from build123d import *

# Parameters (mm, degrees)
SKETCH_1_W                 = 140
SKETCH_1_H                 = 77.4
EXTRUDE_1_DEPTH            = 15
SKETCH_6_R                 = 10.5
CUT_EXTRUDE_4_DEPTH        = 161.315345491
M5X0_8_1_D                 = 4.2
M5X0_8_1_DEPTH             = 16
M5X0_8_1_TIP               = 1.2618073
SKETCH_9_R                 = 10
CUT_EXTRUDE_6_DEPTH        = 161.67283529
M5X0_8_2_D                 = 4.2
HOLE_WIZARD_M3_1_D         = 3.4
M6X1_0_START               = -77.4
M6X1_0_3_OUTLINE_R         = 2.5
M6X1_0_3_DEPTH             = 77.4
HOLE_WIZARD_M3_2_OUTLINE_R = 1.7
HOLE_WIZARD_M3_2_DEPTH     = 15
M7X1_0_4_OUTLINE_W         = 3
M7X1_0_4_OUTLINE_H         = 20.46087378
CUT_EXTRUDE_7_REACH        = 137.336
SKETCH_27_R                = 3


# Read off the part's stored shape, not the designer's step: M6x1.0 ねじ穴3, M3 すきま穴2, M7x1.0 ねじ穴4
with BuildPart() as part:
    # ｽｹｯﾁ1 → ﾎﾞｽ - 押し出し1 (new body)
    with BuildSketch(Plane(origin=(0, 0, 0), x_dir=(1, 0, 0), z_dir=(0, 1, 0))):
        with Locations((70, 38.7)):
            Rectangle(SKETCH_1_W, SKETCH_1_H)
    extrude(amount=EXTRUDE_1_DEPTH)

    # ｽｹｯﾁ6 → ｶｯﾄ - 押し出し4 (cut, through all)
    with BuildSketch(Plane(origin=(0, 10.5, 0), x_dir=(1, 0, 0), z_dir=(0, 1, 0))):
        with Locations(Location((110, 30, 0), (0, 0, 270))):
            Circle(SKETCH_6_R)
    extrude(amount=-CUT_EXTRUDE_4_DEPTH, mode=Mode.SUBTRACT)

    # M5x0.8 ねじ穴1
    with Locations(Plane(origin=(140, 0, 0), x_dir=(0, 0, -1), z_dir=(1, 0, 0))):
        with Locations((10.4, 7.5), (67.4, 7.5)):
            Hole(M5X0_8_1_D / 2, depth=M5X0_8_1_DEPTH)
            with Locations((0, 0, -(M5X0_8_1_DEPTH + M5X0_8_1_TIP / 2))):  # 118° drill point
                Cone(0, M5X0_8_1_D / 2, M5X0_8_1_TIP, mode=Mode.SUBTRACT)

    # ｽｹｯﾁ9 → ｶｯﾄ - 押し出し6 (cut, through all)
    with BuildSketch(Plane(origin=(0, 15, 0), x_dir=(1, 0, 0), z_dir=(0, 1, 0))):
        with Locations(Location((30, 30, 0), (0, 0, 270))):
            Circle(SKETCH_9_R)
    extrude(amount=-CUT_EXTRUDE_6_DEPTH, mode=Mode.SUBTRACT)

    # M5x0.8 ねじ穴2 (through all)
    with Locations(Plane(origin=(0, 15, 0), x_dir=(1, 0, 0), z_dir=(0, 1, 0))):
        with Locations((42.991460674, 42.458810119), (17.272077939, 42.727922061), (42.727922061, 17.272077939), (17.541189881, 17.008539326)):
            Hole(M5X0_8_2_D / 2)

    # M3 すきま穴1 (through all)
    with Locations(Plane(origin=(0, 15, 0), x_dir=(1, 0, 0), z_dir=(0, 1, 0))):
        with Locations((119.899494937, 39.899494937), (119.899494937, 20.100505063), (100.100505063, 20.100505063), (100.100505063, 39.899494937)):
            Hole(HOLE_WIZARD_M3_1_D / 2)

    # M6x1.0 ねじ穴3 outline → M6x1.0 ねじ穴3 (cut)
    with BuildSketch(Plane.XY.offset(M6X1_0_START)):
        with Locations((84.5, 7.5)):
            Circle(M6X1_0_3_OUTLINE_R)
    extrude(amount=M6X1_0_3_DEPTH, mode=Mode.SUBTRACT)

    # M3 すきま穴2 outline → M3 すきま穴2 (cut)
    with BuildSketch(Plane(origin=(0, 0, 0), x_dir=(1, 0, 0), z_dir=(0, 1, 0))):
        with Locations((92.5, 73.4)):
            Circle(HOLE_WIZARD_M3_2_OUTLINE_R)
        with Locations((127.5, 73.4)):
            Circle(HOLE_WIZARD_M3_2_OUTLINE_R)
        with Locations((92.5, 4)):
            Circle(HOLE_WIZARD_M3_2_OUTLINE_R)
        with Locations((127.5, 4)):
            Circle(HOLE_WIZARD_M3_2_OUTLINE_R)
    extrude(amount=HOLE_WIZARD_M3_2_DEPTH, mode=Mode.SUBTRACT)

    # M7x1.0 ねじ穴4 outline → M7x1.0 ねじ穴4 (revolve, cut)
    with BuildSketch(Plane(origin=(0, 7.5, -30), x_dir=(0, 1, 0), z_dir=(0, 0, -1))):
        with Locations((1.5, 10.23043689)):
            Rectangle(M7X1_0_4_OUTLINE_W, M7X1_0_4_OUTLINE_H)
    revolve(axis=Axis((0, 7.5, -30), (1, 0, 0)), mode=Mode.SUBTRACT)

    # ｽｹｯﾁ27 → ｶｯﾄ - 押し出し7 (cut, up to next)
    with BuildSketch(Plane.ZY.offset(-30), mode=Mode.PRIVATE) as cut_extrude_7_sk1:
        with Locations((-30, 7.5)):
            Circle(SKETCH_27_R)
    cut_extrude_7_tool1 = extrude(cut_extrude_7_sk1.sketch, amount=-CUT_EXTRUDE_7_REACH, mode=Mode.PRIVATE) & part.part
    add(cut_extrude_7_tool1.solids().sort_by_distance((30, 7.5, -30))[0], mode=Mode.SUBTRACT)


solid = part.part
Build history of the part. All positions in model axes, mm. A direction names the side the tool comes from. Round coordinates to 2 decimals unless told otherwise and drop trailing zeros. Write each loop counter-clockwise with the first axis right and the second up, starting at its lowest first coordinate (ties: lowest second). Pieces come first, ordered by that corner, then holes. Notation, with made-up numbers: M 20,60 L 59,60 A20 ccw 59,79 Z; hole C 16.25,-14.5 d10. An arc over 180 degrees is marked long. Answer in a Markdown table with one row per item.
1. Probe L1, parallel to X at y = 1.25, z = -42.5; L2, parallel to X at y = 12, z = -4; L3, parallel to X at y = 8.75, z = -73.4. List the from-to ranges inside material, lowest first. Write a range as [from, to].
Geometry check:
| item | result |
|---|---|
| L1 | [0, 15.18], [19.36, 40.89], [45.09, 140] |
| L2 | [0, 90.8], [94.2, 125.8], [129.2, 140] |
| L3 | [0, 82.33], [86.67, 90.8], [94.2, 125.8], [129.2, 140] |
2. Saw through at B-B (z = -4). List the corners of the cut face in (x, y), and give its area (3 significant figures).
Geometry check:
| item | result |
|---|---|
| outline | M 0,0 L 90.8,0 L 90.8,15 L 0,15 Z; M 94.2,0 L 125.8,0 L 125.8,15 L 94.2,15 Z; M 129.2,0 L 140,0 L 140,15 L 129.2,15 Z; hole C 84.5,7.5 d5 |
| area | 1,980 mm2 |
3. Saw through at D-D (z = -35). List the corners of the cut face in (x, y).
Geometry check:
| item | result |
|---|---|
| outline | M 0,0 L 21.34,0 L 21.34,15 L 0,15 Z; M 38.66,0 L 100.77,0 L 100.77,10.5 L 119.23,10.5 L 119.23,0 L 140,0 L 140,15 L 38.66,15 Z; hole C 84.5,7.5 d5 |
4. Which spindle directions (+Z, -Z, +X, -X, +Y, -Y) get a long thin tool onto all of the face, cutting with end or side? Do faces 1 (the face through (10.38, 10.27, -31.15)), 2 (the face through (120.41, 5.32, -31.37)), 3 (the face through (131.888, 9.582, -10.673)). Say none if no direction does.
Geometry check:
| item | result |
|---|---|
| face 1 | -X |
| face 2 | -Y |
| face 3 | +X |
5. Mould opens along Z. For faces 4 (the face through (69, 0, -39)), 5 (the face through (44.826, 7.395, -17.364)) say: +Z half, -Z half, draft (parallel to the pull), parting line (faces both ways), or undercut.
Geometry check:
| item | result |
|---|---|
| face 4 | draft |
| face 5 | undercut |
6. Flat gauge pins, fed straight in: P1, Ø4, axis at y = 7.5, z = -67.4, coming from the +X side; P2, Ø5.5, axis at y = 7.5, z = -30, coming from the -X side. Where does each tip first touch, or does it go through?
Geometry check:
| item | result |
|---|---|
| P1 | x = 123.94 |
| P2 | x = 120.13 |
7. Saw through at C-C (x = 43). List the corners of the cut face in (y, z), and give its area (3 significant figures).
Geometry check:
| item | result |
|---|---|
| outline | M 0,-77.4 L 15,-77.4 L 15,-44.56 L 0,-44.56 Z; M 0,-40.36 L 15,-40.36 L 15,-19.35 L 0,-19.35 Z; M 0,-15.19 L 15,-15.19 L 15,0 L 0,0 Z; hole C 7.5,-30 d6 |
| area | 1,010 mm2 |
8. Saw through at A-A (x = 127.5). List the corners of the cut face in (y, z).
Geometry check:
| item | result |
|---|---|
| outline | M 0,-77.4 L 15,-77.4 L 15,-75.1 L 0,-75.1 Z; M 0,-71.7 L 15,-71.7 L 15,-5.7 L 0,-5.7 Z; M 0,-2.3 L 15,-2.3 L 15,0 L 0,0 Z; hole C 7.5,-67.4 d4.2; hole C 7.5,-10.4 d4.2 |
